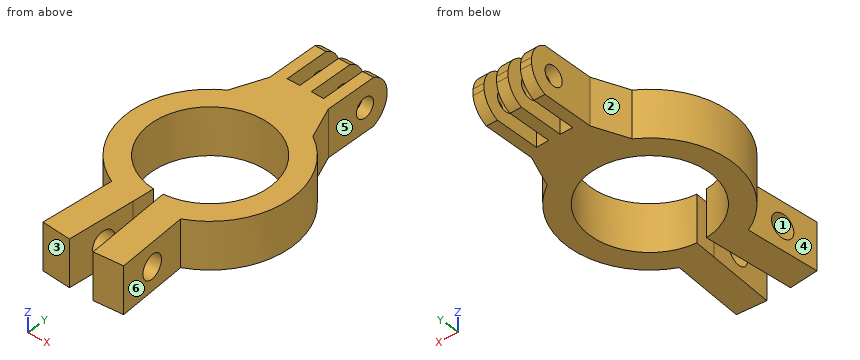
```python
from build123d import *

# Parameters (mm, degrees)
F1_DEPTH = 13
F3_DEPTH = 17
F2_R     = 2.7179879064
F4_DEPTH = 17
F5_R     = 3.25
F6_DEPTH = 13
F7_R     = 3.25
F8_DEPTH = 13


with BuildPart() as f1:
    # F0 (on Top) → F1 (new body)
    with BuildSketch(Plane.XY):
        with BuildLine():
            Line((11.2865111771, -40.2498981271), (9.6717664856, -20.3151897123))
            ThreePointArc((9.6717664856, -20.3151897123), (22.4638141096, -1.275560915), (11.9092941804, 19.0897541138))
            ThreePointArc((11.9092941804, 19.0897541138), (10.094643898, 20.1084102945), (8.1936409697, 20.955053034))
            ThreePointArc((8.1936409697, 20.955053034), (0, 22.5), (-8.1936409697, 20.955053034))
            ThreePointArc((-8.1936409697, 20.955053034), (-10.094643898, 20.1084102945), (-11.9092941804, 19.0897541138))
            ThreePointArc((-11.9092941804, 19.0897541138), (-22.4638141096, -1.275560915), (-9.6717664856, -20.3151897123))
            Line((-9.6717664856, -20.3151897123), (-11.2865111771, -40.2498981271))
            Line((-11.2865111771, -40.2498981271), (-3.3126278112, -40.8957960037))
            Line((-3.3126278112, -40.8957960037), (-1.816587778, -22.4265469666))
            Line((-1.816587778, -22.4265469666), (-1.3321643705, -16.4461344422))
            ThreePointArc((-1.3321643705, -16.4461344422), (0, 16.5), (1.3321643705, -16.4461344422))
            Line((1.3321643705, -16.4461344422), (1.816587778, -22.4265469666))
            Line((1.816587778, -22.4265469666), (3.3126278112, -40.8957960037))
            Line((3.3126278112, -40.8957960037), (11.2865111771, -40.2498981271))
        make_face()
        with BuildLine():
            ThreePointArc((8.1936409697, 20.955053034), (10.094643898, 20.1084102945), (11.9092941804, 19.0897541138))
            Line((11.9092941804, 19.0897541138), (8.1936409697, 28.2182842493))
            Line((8.1936409697, 28.2182842493), (8.1936409697, 20.955053034))
        make_face()
        with BuildLine():
            ThreePointArc((-8.1936409697, 20.955053034), (0, 22.5), (8.1936409697, 20.955053034))
            Line((8.1936409697, 20.955053034), (8.1936409697, 28.2182842493))
            Line((8.1936409697, 28.2182842493), (8.1936409697, 46.824157238))
            Line((8.1936409697, 46.824157238), (5.0982660614, 46.824157238))
            Line((5.0982660614, 46.824157238), (5.0982660614, 30.2175015012))
            Line((5.0982660614, 30.2175015012), (1.6, 30.2903222447))
            Line((1.6, 30.2903222447), (1.6, 46.824157238))
            Line((1.6, 46.824157238), (0, 46.824157238))
            Line((0, 46.824157238), (-1.6, 46.824157238))
            Line((-1.6, 46.824157238), (-1.6, 30.2903222447))
            Line((-1.6, 30.2903222447), (-5.0982660614, 30.2175015012))
            Line((-5.0982660614, 30.2175015012), (-5.0982660614, 46.824157238))
            Line((-5.0982660614, 46.824157238), (-8.1936409697, 46.824157238))
            Line((-8.1936409697, 46.824157238), (-8.1936409697, 33.1387296319))
            Line((-8.1936409697, 33.1387296319), (-8.1936409697, 28.2182842493))
            Line((-8.1936409697, 28.2182842493), (-8.1936409697, 20.955053034))
        make_face()
        with BuildLine():
            ThreePointArc((-11.9092941804, 19.0897541138), (-10.094643898, 20.1084102945), (-8.1936409697, 20.955053034))
            Line((-8.1936409697, 20.955053034), (-8.1936409697, 28.2182842493))
            Line((-8.1936409697, 28.2182842493), (-11.9092941804, 19.0897541138))
        make_face()
    extrude(amount=F1_DEPTH)

    # F2 (on face) → F3 (cut)
    with BuildSketch(Plane.YZ.offset(8.1936409697)):
        with BuildLine():
            ThreePointArc((42.5635200859, 13), (45.44932769, 10.755768579), (46.824157238, 7.3683943876))
            Line((46.824157238, 7.3683943876), (46.824157238, 13))
            Line((46.824157238, 13), (42.5635200859, 13))
        make_face()
        with BuildLine():
            Line((46.824157238, 0), (46.824157238, 5.6316056124))
            ThreePointArc((46.824157238, 5.6316056124), (45.44932769, 2.244231421), (42.5635200859, 0))
            Line((42.5635200859, 0), (46.824157238, 0))
        make_face()
    extrude(amount=-F3_DEPTH, mode=Mode.SUBTRACT)

    # F2 (on face) → F4 (cut)
    with BuildSketch(Plane.YZ.offset(8.1936409697)):
        with Locations((39.824157238, 6.5)):
            Circle(F2_R)
    extrude(amount=-F4_DEPTH, mode=Mode.SUBTRACT)

    # F5 (on face) → F6 (cut)
    with BuildSketch(Plane(origin=(7.9738833659, 0.6458978766, 0), x_dir=(-0.0807372346, 0.9967354207, 0), z_dir=(0.9967354207, 0.0807372346, 0))):
        with Locations((-31.0297408448, 6.5)):
            Circle(F5_R)
    extrude(amount=-F6_DEPTH, mode=Mode.SUBTRACT)

    # F7 (on face) → F8 (cut)
    with BuildSketch(Plane(origin=(-7.9738833659, 0.6458978766, 0), x_dir=(-0.0807372346, -0.9967354207, 0), z_dir=(-0.9967354207, 0.0807372346, 0))):
        with Locations((31.0297408448, 6.5)):
            Circle(F7_R)
    extrude(amount=-F8_DEPTH, mode=Mode.SUBTRACT)


solid = f1.part
```
Design review of the part built by this model. Coordinates are the model's own, in mm. Face numbers are marked on the shaded views. A direction names the side the tool comes from. Coordinates: 2 decimals unless noted, no trailing zeros. Order: outer loops, then holes, each group sorted by start corner. A loop starts at its lowest first (then second) coordinate and runs counter-clockwise, first axis right, second up. Notation, with made-up numbers: (82.25, 38) - (122.25, 38) arc R32 cw to (122.25, 67) - close; hole circle Ø4 at (-5.5, 42). An arc over 180 degrees is marked (long way). One line per question, with ' | ' between items.
Q1. Consider section C-C, the plane x = -13. Give the boundary of the cut face in (y, z).
Answer key:
outline: (-18.36, 0) - (-10.16, 0) - (-10.16, 13) - (-18.36, 13) - close; (10.16, 0) - (18.36, 0) - (18.36, 13) - (10.16, 13) - close
Q2. Consider section D-D, the plane z = 2. Give the boundary of the cut face in (x, y).
Answer key:
outline: (-11.91, 19.09) arc R22.5 ccw to (-9.67, -20.32) - (-11.29, -40.25) - (-3.31, -40.9) - (-1.33, -16.45) arc R16.5 cw (long way) to (1.33, -16.45) - (3.31, -40.9) - (11.29, -40.25) - (9.67, -20.32) arc R22.5 ccw to (11.91, 19.09) - (8.19, 28.22) - (8.19, 45.26) - (5.1, 45.26) - (5.1, 30.22) - (1.6, 30.29) - (1.6, 45.26) - (-1.6, 45.26) - (-1.6, 30.29) - (-5.1, 30.22) - (-5.1, 45.26) - (-8.19, 45.26) - (-8.19, 28.22) - close
Q3. For the marked faces 4, 5 and 6, list the 3-axis set-ups (+Z, -Z, +X, -X, +Y, -Y) from which the entire face can be reached by the end or side of a thin tool; tool diameter is ignored.
Answer key:
face 4: +Z, -Z, -X | face 5: +Z, -Z, +X, +Y | face 6: +Z, -Z, +X
Q4. To check wall thickness, follow line 1 along X through (y, z) = (35.5, 0.5); line 2 along X through (y, z) = (0, 6.5); line 3 along Y through (x, z) = (-9.5, 9.5). State the ranges of each line that lie inside material, in increasing order.
Answer key:
line 1: x = -8.19 to -5.1, -1.6 to 1.6, 5.1 to 8.19 | line 2: x = -22.5 to -16.5, 16.5 to 22.5 | line 3: y = -40.39 to -31.62, -29.11 to -13.49, 13.49 to 25.01
Q5. Clearance check with flat-ended pins moving along their axes: pin 1 Ø4 at (y, z) = (-7.5, 6) entering from -X; pin 2 Ø4 at (y, z) = (34.5, 8) entering from -X; pin 3 Ø6.5 at (y, z) = (39.82, 6.5) entering from +X; pin 4 Ø8 at (x, y) = (11.5, -20) entering from +Z. State where each tip first meets the part, or that it passes through.
Answer key:
pin 1: stops at x = -21.82 | pin 2: stops at x = -8.19 | pin 3: stops at x = 8.19 | pin 4: stops at z = 13
Q6. The part is to be moulded in two halves that separate along Y. For the marked faces 1, 2 and 3, say which applies: +Y half, -Y half, draft (parallel to the pull), parting line (faces both ways), or undercut.
Answer key:
face 1: undercut | face 2: +Y half | face 3: -Y half
Q7. Consider section A-A, the plane x = 0. Give the boundary of the cut face in (y, z).
Answer key:
outline: (16.5, 0) - (42.56, 0) arc R7.05 ccw to (46.82, 5.63) - (46.82, 7.37) arc R7.05 ccw to (42.56, 13) - (16.5, 13) - close; hole circle Ø5.44 at (39.82, 6.5)
Q8. Consider section B-B, the plane y = 0. Give the boundary of the cut face in (x, z), then the cut area to 3 significant figures.
Answer key:
outline: (-22.5, 0) - (-16.5, 0) - (-16.5, 13) - (-22.5, 13) - close; (16.5, 0) - (22.5, 0) - (22.5, 13) - (16.5, 13) - close | area: 156 mm2
